Could you check a few things on this model? Use its own coordinates, in mm. A direction names the side the tool comes from. Give positions to 0.01 mm unless a question says otherwise; leave off trailing zeros. Loops run counter-clockwise (first coordinate to the right, second up) from the corner with the lowest first, then second, coordinate; pieces in that order, holes last. Notation, with made-up numbers: (61, 43.5) -> (95, 43.5) arc R8 cw to (95, 56.5) -> close; hole circle Ø5 at (46, 80.25). An arc over 180 degrees is marked (long way). Put each result on its own line as item: value.
```python
from build123d import *

# Parameters (mm, degrees)
BASE_FLANGE1_DEPTH = 10
FILLET1_R          = 3
SKETCH6_R          = 1.5
CUT_EXTRUDE1_DEPTH = 18.549928775
SKETCH7_R          = 0.75
CUT_EXTRUDE2_DEPTH = 18.549928775


# Sheet-metal steps are written as plain solids
with BuildPart() as part:
    # Sketch1 → Base-Flange1 (new, symmetric)
    with BuildSketch(Plane.XY):
        with BuildLine():
            Line((-12, 0), (-0.75, 0))
            ThreePointArc((-0.75, 0), (-0.219669914, 0.219669914), (0, 0.75))
            Line((0, 0.75), (0, 8))
            Line((0, 8), (2, 8))
            Line((2, 8), (2, 0.75))
            ThreePointArc((2, 0.75), (1.194543648, -1.194543648), (-0.75, -2))
            Line((-0.75, -2), (-12, -2))
            Line((-12, -2), (-12, 0))
        make_face()
    extrude(amount=BASE_FLANGE1_DEPTH, both=True)

    # Fillet1
    fillet1_edges = [part.edges().sort_by_distance(p)[0] for p in [
        (-12, -1, 10),
        (-12, -1, -10),
        (1, 8, 10),
        (1, 8, -10),
    ]]
    fillet(fillet1_edges, radius=FILLET1_R)

    # Sketch6 → Cut-Extrude1 (cut, through all)
    with BuildSketch(Plane(origin=(0, 0, 0), x_dir=(1, 0, 0), z_dir=(0, 1, 0))):
        with Locations(Location((-9, 6, 0), (0, 0, 270))):
            Circle(SKETCH6_R)
        with Locations(Location((-9, -6, 0), (0, 0, 90))):
            Circle(SKETCH6_R)
    extrude(amount=-CUT_EXTRUDE1_DEPTH, mode=Mode.SUBTRACT)

    # Sketch7 → Cut-Extrude2 (cut, through all)
    with BuildSketch(Plane.ZY):
        with Locations((0, 6)):
            Circle(SKETCH7_R)
    extrude(amount=-CUT_EXTRUDE2_DEPTH, mode=Mode.SUBTRACT)


solid = part.part
```
1. If we section it at C-C (y = 6): List the corners of the cut face in (x, z) for me, then the cut area to 3 significant figures.
Recorded:
outline: (0, -9.83) -> (2, -9.83) -> (2, -0.75) -> (0, -0.75) -> close; (0, 0.75) -> (2, 0.75) -> (2, 9.83) -> (0, 9.83) -> close
area: 36.3 mm^2
2. If we section it at B-B (z = 6): List the corners of the cut face in (x, y) for me, then the cut area to 3 significant figures.
Recorded:
outline: (-12, -2) -> (-10.5, -2) -> (-10.5, 0) -> (-12, 0) -> close; (-7.5, -2) -> (-0.75, -2) arc R2.75 ccw to (2, 0.75) -> (2, 8) -> (0, 8) -> (0, 0.75) arc R0.75 cw to (-0.75, 0) -> (-7.5, 0) -> close
area: 36.5 mm^2
3. I'm going to push flat-ended pins straight in: pin 1 (5.5 mm diameter, centred on x = -7.5, z = 4, fed in from +Y); pin 2 (1.2 mm diameter, centred on y = 6, z = 0, fed in from +X); pin 3 (4 mm diameter, centred on y = 7, z = -6, fed in from -X). Where does each tip first touch, or does it pass through?
Recorded:
pin 1: stops at y = 0
pin 2: passes through
pin 3: stops at x = 0
4. Thinking about a two-plate mould opening in Z: for faces 1 (the face through (-10.464, -0.986, -6.325)), 2 (the face through (-12, -1, 0)), 3 (the face through (-11.1, -0.99, -9.14)), which applies, pulls with the +Z half, pulls with the -Z half, needs draft (parallel to the pull), parting line crosses it, or undercut?
Recorded:
face 1: undercut
face 2: needs draft
face 3: pulls with the -Z half
5. I need wall thicknesses on line 1 (X direction, y = -0.9, z = -6); line 2 (X direction, y = 1, z = -0.5); line 3 (Y direction, x = 0.5, z = 0). Which ranges of each line are inside material? Lowest first, please.
Recorded:
line 1: x = -12 to -10.5, -7.5 to 1.45
line 2: x = 0 to 2
line 3: y = -1.7 to 5.25, 6.75 to 8
6. If we section it at A-A (z = 0): List the corners of the cut face in (x, y) for me.
Recorded:
outline: (-12, -2) -> (-0.75, -2) arc R2.75 ccw to (2, 0.75) -> (2, 5.25) -> (0, 5.25) -> (0, 0.75) arc R0.75 cw to (-0.75, 0) -> (-12, 0) -> close; (0, 6.75) -> (2, 6.75) -> (2, 8) -> (0, 8) -> close
7. For faces 4 (the face through (0, 4, 0)), 5 (the face through (0.986, 5.268, -0.163)), which set-ups out of +Z, -Z, +X, -X, +Y, -Y let a thin tool reach every point of the face, with its end or its side?
Recorded:
face 4: +Z, -Z, -X, +Y
face 5: +X, -X
8. If we section it at D-D (y = -0.5): List the corners of the cut face in (x, z) for me, then the cut area to 3 significant figures.
Recorded:
outline: (-12, -7) arc R3 ccw to (-9, -10) -> (1.7, -10) -> (1.7, 10) -> (-9, 10) arc R3 ccw to (-12, 7) -> close; hole circle Ø3 at (-9, -6); hole circle Ø3 at (-9, 6)
area: 256 mm^2
